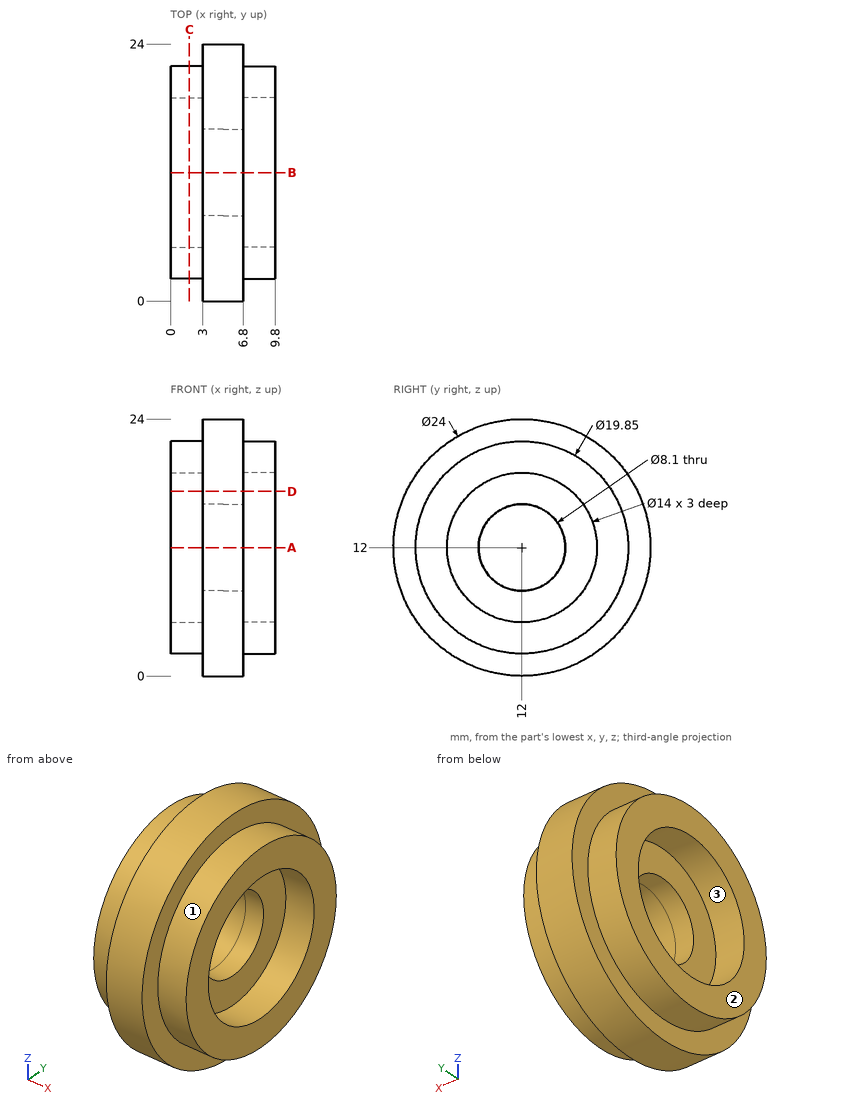
Here's the drawing with two shaded views (mm, measured from the low corner). I have some questions. A direction names the side the tool comes from. Coordinates: 2 decimals unless noted, no trailing zeros. Write each loop counter-clockwise with the first axis right and the second up, starting at its lowest first coordinate (ties: lowest second). Pieces come first, ordered by that corner, then holes. Notation, with made-up numbers: (73.5, -22.75) -> (121.5, -22.75) arc R9 ccw to (121.5, -16.75) -> close; hole circle Ø6 at (42, 19). An arc over 180 degrees is marked (long way). One line per question, with ' | ' between items. Start each with the question number.
1. If we section it at C-C (x = 1.75): Please give me the cut outline in (y, z) (3 decimals).
2. For the marked faces 1, 2 and 3, which set-ups out of +Z, -Z, +X, -X, +Y, -Y let a thin tool reach every point of the face, with its end or its side?
3. Please list where these lines run through material, in increasing order: line 1 along Y through (x, z) = (0.85, 12) (3 decimals); line 2 along Y through (x, z) = (5.9, 12); line 3 along X through (y, z) = (13.75, 16.75).
4. If we section it at D-D (z = 17.25): Please give me the cut outline in (x, y).
5. If we section it at A-A (z = 12): Please give me the cut outline in (x, y) (3 decimals), and give its area (3 significant figures).
6. Will these pins go through, and if not, where does the flat tip stop? P1, Ø4, axis at y = 15.5, z = 15, coming from the -X side; P2, Ø5, axis at x = 8.5, y = 16.5, coming from the +Z side; P3, Ø12.5, axis at y = 12, z = 12, coming from the +X side.
Return value:
1) outline: circle Ø19.85 at (12, 12); hole circle Ø14 at (12, 12)
2) face 1: +X | face 2: +Z, -Z, -X, +Y, -Y | face 3: -X
3) line 1: y = 2.075 to 5, 19 to 21.925 | line 2: y = 0 to 7.95, 16.05 to 24 | line 3: x = 3 to 6.8
4) outline: (0, 3.58) -> (3, 3.58) -> (3, 1.21) -> (6.8, 1.21) -> (6.8, 3.58) -> (9.8, 3.58) -> (9.8, 7.37) -> (6.8, 7.37) -> (6.8, 16.63) -> (9.8, 16.63) -> (9.8, 20.42) -> (6.8, 20.42) -> (6.8, 22.79) -> (3, 22.79) -> (3, 20.42) -> (0, 20.42) -> (0, 16.63) -> (3, 16.63) -> (3, 7.37) -> (0, 7.37) -> close
5) outline: (0, 2.075) -> (3, 2.075) -> (3, 0) -> (6.8, 0) -> (6.8, 2.075) -> (9.8, 2.075) -> (9.8, 5) -> (6.8, 5) -> (6.8, 7.95) -> (3, 7.95) -> (3, 5) -> (0, 5) -> close; (0, 19) -> (3, 19) -> (3, 16.05) -> (6.8, 16.05) -> (6.8, 19) -> (9.8, 19) -> (9.8, 21.925) -> (6.8, 21.925) -> (6.8, 24) -> (3, 24) -> (3, 21.925) -> (0, 21.925) -> close | area: 95.5 mm²
6) P1: stops at x = 3 | P2: stops at z = 23.7 | P3: stops at x = 6.8
